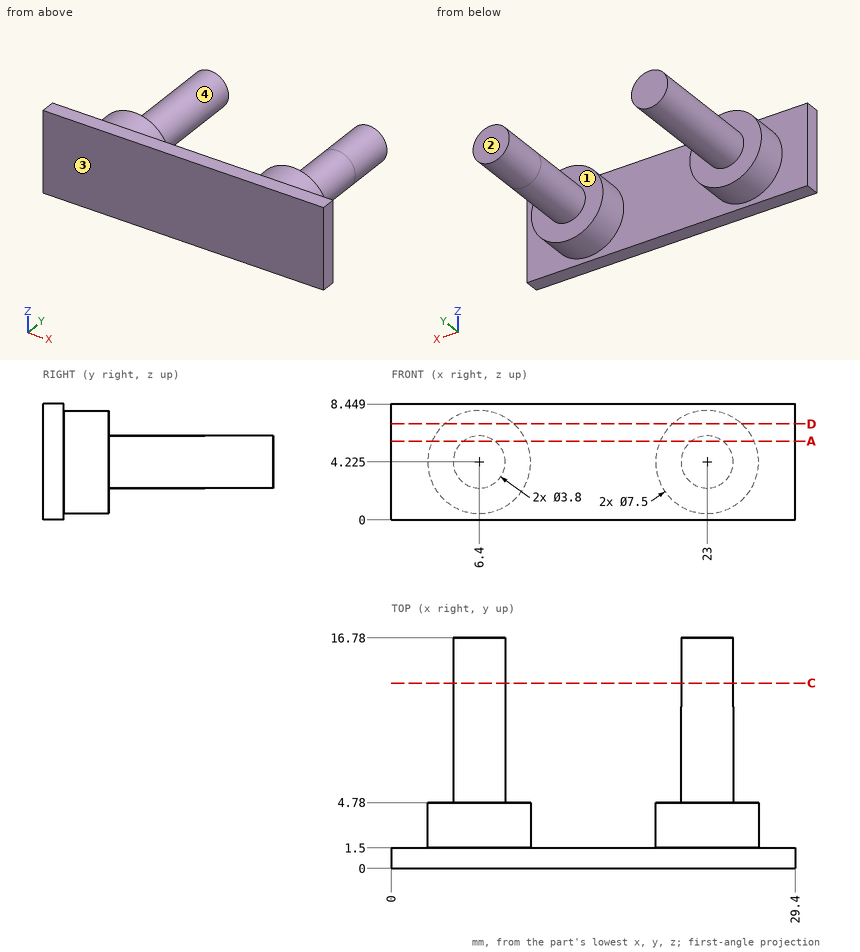
The drawing under review shows one solid part. Ordinate dimensions are in mm from its lowest x, y, z. A direction names the side the tool comes from. Coordinates: 2 decimals unless noted, no trailing zeros. Write each loop counter-clockwise with the first axis right and the second up, starting at its lowest first coordinate (ties: lowest second). Pieces come first, ordered by that corner, then holes.
1) Mouldability with a two-part tool opening along X and no side actions: class the marked faces 3 and 4 as +X half, -X half, draft (parallel to the pull), parting line (faces both ways), or undercut.
2) Add section C-C (y = 13.5). Write out the cut boundary in (x, z) (1 decimal).
3) Insertion check: pin 1 (1 mm diameter, centred on y = 11, z = 1.5, fed in from +X); pin 2 (5 mm diameter, centred on y = 7, z = 1, fed in from +X) (1 decimal); pin 3 (4 mm diameter, centred on x = 4, z = 1, fed in from +Y). Each pin has a flat end and moves straight along its axis. Give the tip position at first contact, or say it passes through.
4) To check wall thickness, follow L1, parallel to Y at x = 15.75, z = 6; L2, parallel to X at y = 4, z = 7.5 (1 decimal); L3, parallel to Y at x = 22.75, z = 1. State the ranges of each line that lie inside material, in increasing order.
5) Add section D-D (z = 7). Write out the cut boundary in (x, y).
6) Machinability: for the marked faces 1 and 2, which of the approach directions +Z, -Z, +X, -X, +Y, -Y give a long, thin tool a straight path to every point of the face, cutting with its end or side? Answer none if there is none.
7) Add section A-A (z = 5.75). Write out the cut boundary in (x, y) (1 decimal).
Check result:
1. face 3: draft
1. face 4: undercut
2. outline: circle Ø3.8 at (6.4, 4.2); circle Ø3.8 at (23, 4.2)
3. pin 1: passes through
3. pin 2: stops at x = 26.1
3. pin 3: stops at y = 4.78
4. L1: y = 0 to 1.5
4. L2: x = 4.6 to 8.2, 21.2 to 24.8
4. L3: y = 0 to 4.78
5. outline: (0, 0) - (29.4, 0) - (29.4, 1.5) - (25.52, 1.5) - (25.52, 4.78) - (20.48, 4.78) - (20.48, 1.5) - (8.92, 1.5) - (8.92, 4.78) - (3.88, 4.78) - (3.88, 1.5) - (0, 1.5) - close
6. face 1: +Y
6. face 2: +Z, -Z, +X, -X, +Y
7. outline: (0, 0) - (29.4, 0) - (29.4, 1.5) - (26.4, 1.5) - (26.4, 4.8) - (24.1, 4.8) - (24.1, 16.8) - (21.9, 16.8) - (21.9, 4.8) - (19.6, 4.8) - (19.6, 1.5) - (9.8, 1.5) - (9.8, 4.8) - (7.5, 4.8) - (7.5, 16.8) - (5.3, 16.8) - (5.3, 4.8) - (3, 4.8) - (3, 1.5) - (0, 1.5) - close
